Geometry: see drawing. Coordinates: mm, zero at the bounding-box minimum. A direction names the side the tool comes from. Give positions to 0.01 mm unless a question says otherwise; leave off trailing zeros. Order: outer loops, then holes, each group sorted by start corner. A loop starts at its lowest first (then second) coordinate and runs counter-clockwise, first axis right, second up. Notation, with made-up numbers: M 60.25,77.25 L 85.25,77.25 A17 cw 85.25,103.25 Z; hole C 52.5,0 d11. An arc over 180 degrees is marked long. Answer as a JSON object with one key per item and string values. Group by question number.
1. Section query A-A (y = 16). Output: boundary loops of the cut face in (x, z) (3 decimals), plus the area to 3 significant figures.
2. Section query D-D (z = 6). Output: boundary loops of the cut face in (x, y), plus the area to 3 significant figures.
3. Pull-direction query (X, two-part tool) for the marked faces 1, 2 and 3; classes: +X half, -X half, draft (parallel to the pull), parting line (faces both ways), or undercut.
4. Set-up query: the marked faces 4, 5 and 6. Return all of +Z, -Z, +X, -X, +Y, -Y with unobstructed straight access to the full face (end or side cutting, diameter ignored); none if empty.
5. Section query B-B (x = 27.5). Output: boundary loops of the cut face in (y, z).
6. Section query C-C (z = 3.5). Output: boundary loops of the cut face in (x, y) (3 decimals).
7. Material intervals for L1, parallel to X at y = 4, z = 2; L2, parallel to X at y = 25.5, z = 3.25; L3, parallel to X at y = 4.5, z = 4, sorted ascending. Write a range as [from, to].
8. Pin query (flat end, axial travel): P1, Ø3.5, axis at x = 34.5, z = 3.5, coming from the -Y side. Return the tip coordinate at first contact, or that it passes through.
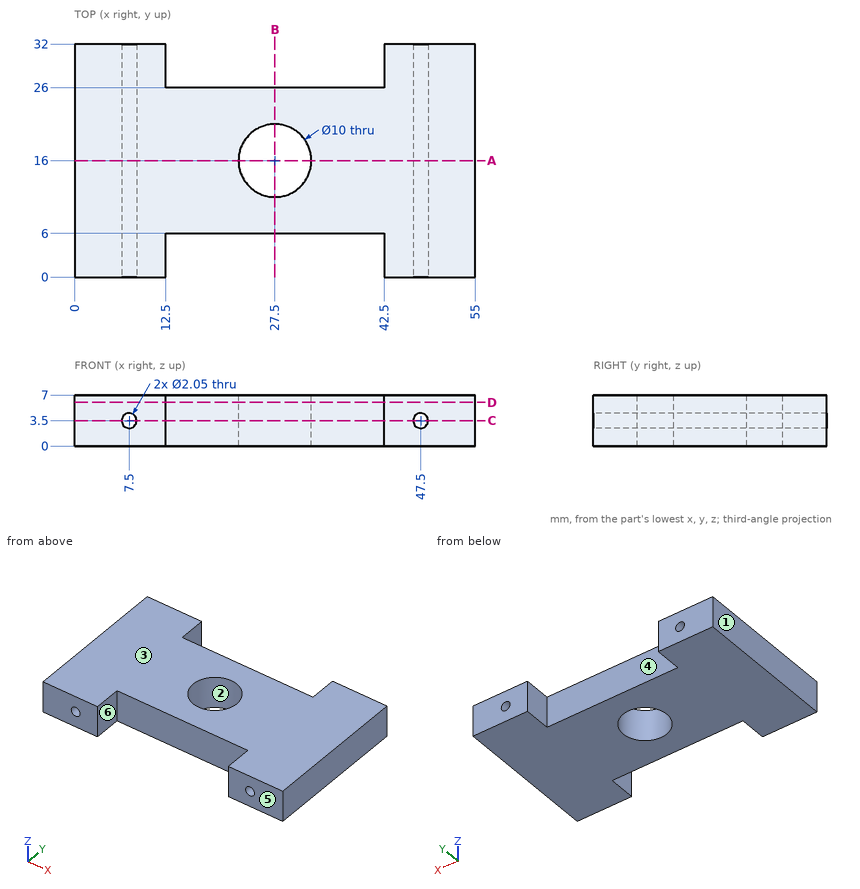
Answer sheet:
{
 "1": {"outline": "M 0,0 L 22.5,0 L 22.5,7 L 0,7 Z; M 32.5,0 L 55,0 L 55,7 L 32.5,7 Z; hole C 7.5,3.5 d2.05; hole C 47.5,3.5 d2.05", "area": "308 mm^2"},
 "2": {"outline": "M 0,0 L 12.5,0 L 12.5,6 L 42.5,6 L 42.5,0 L 55,0 L 55,32 L 42.5,32 L 42.5,26 L 12.5,26 L 12.5,32 L 0,32 Z; hole C 27.5,16 d10", "area": "1,320 mm^2"},
 "3": {"face 1": "-X half", "face 2": "undercut", "face 3": "draft"},
 "4": {"face 4": "+Z, -Z, +Y", "face 5": "+Z, -Z, +X, -X, -Y", "face 6": "+Z, -Z, -Y"},
 "5": {"outline": "M 6,0 L 11,0 L 11,7 L 6,7 Z; M 21,0 L 26,0 L 26,7 L 21,7 Z"},
 "6": {"outline": "M 0,0 L 6.475,0 L 6.475,32 L 0,32 Z; M 8.525,0 L 12.5,0 L 12.5,6 L 42.5,6 L 42.5,0 L 46.475,0 L 46.475,32 L 42.5,32 L 42.5,26 L 12.5,26 L 12.5,32 L 8.525,32 Z; M 48.525,0 L 55,0 L 55,32 L 48.525,32 Z; hole C 27.5,16 d10"},
 "7": {"L1": "[0, 12.5], [42.5, 55]", "L2": "[0, 6.51], [8.49, 46.51], [48.49, 55]", "L3": "[0, 6.61], [8.39, 12.5], [42.5, 46.61], [48.39, 55]"},
 "8": {"P1": "y = 6"}
}
